Input: dimensioned drawing with shaded views. Units: mm. Origin: part minimum x, y, z. A direction names the side the tool comes from. Give positions to 0.01 mm unless a question says otherwise; leave off trailing zeros. Write each loop counter-clockwise with the first axis right and the second up, starting at its lowest first coordinate (ties: lowest second). Pieces come first, ordered by that corner, then holes. Notation, with made-up numbers: (-6.75, 72) -> (45.25, 72) arc R37 cw to (45.25, 110) -> close; hole circle Ø10 at (-2.75, 59.25). An arc over 180 degrees is marked (long way). Answer as a JSON object with one key per item and string values. Group by question number.
(1) Set-up query: the marked faces 5 and 6. Return all of +Z, -Z, +X, -X, +Y, -Y with unobstructed straight access to the full face (end or side cutting, diameter ignored); none if empty.
(2) Draft query along Z for the marked faces 1, 2, 3 and 4. Return one class per face: +Z half, -Z half, draft (parallel to the pull), parting line (faces both ways), or undercut.
(3) Section query C-C on y = 2.3. Output: boundary loops of the cut face in (x, z), plus the area to 3 significant figures.
(4) Contact query for flat-ended pins moving along their axis: pin 1 Ø3 at (x, z) = (9.75, 16.75) entering from +Y; pin 2 Ø1 at (x, y) = (7.5, 1) entering from -Z; pin 3 Ø1.5 at (x, y) = (7, 4.5) entering from +Z. Output: stop coordinate, or through.
(5) Section query B-B on x = 8.75. Output: boundary loops of the cut face in (y, z), plus the area to 3 significant figures.
(6) Section query D-D on x = 17.75. Output: boundary loops of the cut face in (y, z), plus the area to 3 significant figures.
(7) Section query A-A on z = 15.75. Output: boundary loops of the cut face in (x, y).
(8) Material intervals for probe 1 along X at (y, z) = (0.55, 9.75); probe 2 along X at (y, z) = (1.85, 9.75); probe 3 along Y at (x, z) = (16.5, 5), sorted ascending.
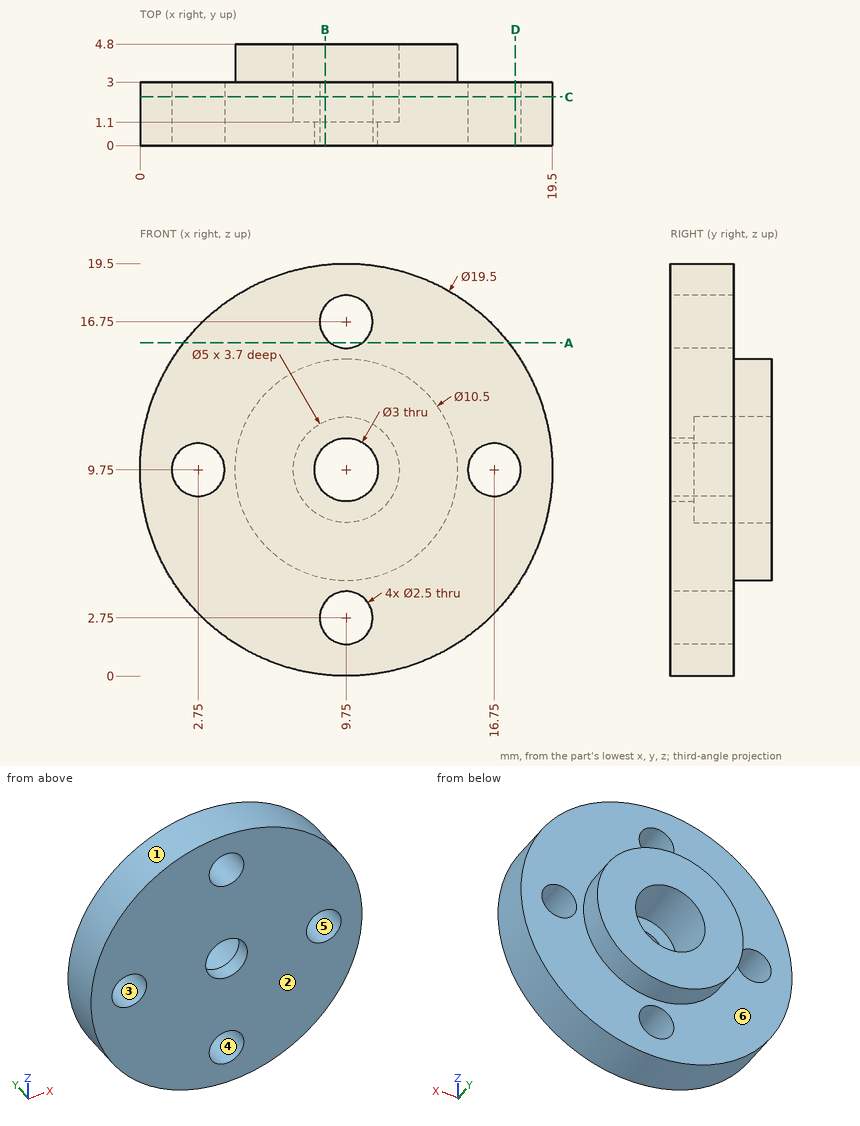
Answer list:
{
 "1": {"face 5": "+Y, -Y", "face 6": "+Y"},
 "2": {"face 1": "parting line", "face 2": "draft", "face 3": "undercut", "face 4": "undercut"},
 "3": {"outline": "circle Ø19.5 at (9.75, 9.75); hole circle Ø2.5 at (2.75, 9.75); hole circle Ø5 at (9.75, 9.75); hole circle Ø2.5 at (9.75, 2.75); hole circle Ø2.5 at (9.75, 16.75); hole circle Ø2.5 at (16.75, 9.75)", "area": "259 mm2"},
 "4": {"pin 1": "y = 3", "pin 2": "z = 0.16", "pin 3": "z = 14.6"},
 "5": {"outline": "(0, 0.05) -> (3, 0.05) -> (3, 2) -> (0, 2) -> close; (0, 3.5) -> (3, 3.5) -> (3, 4.6) -> (4.8, 4.6) -> (4.8, 7.46) -> (1.1, 7.46) -> (1.1, 8.63) -> (0, 8.63) -> close; (0, 10.87) -> (1.1, 10.87) -> (1.1, 12.04) -> (4.8, 12.04) -> (4.8, 14.9) -> (3, 14.9) -> (3, 16) -> (0, 16) -> close; (0, 17.5) -> (3, 17.5) -> (3, 19.45) -> (0, 19.45) -> close", "area": "48.3 mm2"},
 "6": {"outline": "(0, 4.18) -> (3, 4.18) -> (3, 9) -> (0, 9) -> close; (0, 10.5) -> (3, 10.5) -> (3, 15.32) -> (0, 15.32) -> close", "area": "28.9 mm2"},
 "7": {"outline": "(2.06, 0) -> (9, 0) -> (9, 3) -> (2.06, 3) -> close; (10.5, 0) -> (17.44, 0) -> (17.44, 3) -> (10.5, 3) -> close"},
 "8": {"probe 1": "0 to 1.5, 4 to 8.25, 11.25 to 15.5, 18 to 19.5", "probe 2": "0 to 1.5, 4 to 7.25, 12.25 to 15.5, 18 to 19.5", "probe 3": "0 to 3"}
}
